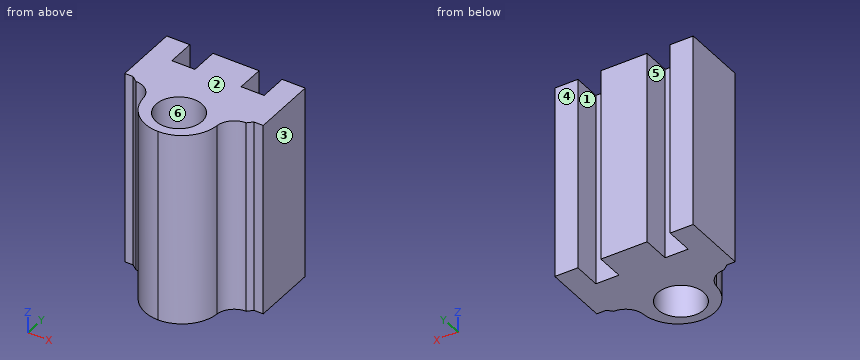
from build123d import *

# Parameters (mm, degrees)
SKETCH1_W           = 60
SKETCH1_H           = 42
BOSS_EXTRUDE1_DEPTH = 8
SKETCH3_W           = 10
SKETCH3_H           = 42
BOSS_EXTRUDE5_DEPTH = 6
SKETCH5_W           = 14
SKETCH5_H           = 42
BOSS_EXTRUDE6_DEPTH = 11
SKETCH6_R           = 5
CUT_EXTRUDE1_DEPTH  = 75.565407529
FILLET1_R           = 7
FILLET2_R           = 5
FILLET3_R           = 5
BOSS_EXTRUDE7_DEPTH = 42
SKETCH9_W           = 5
SKETCH9_H           = 42
BOSS_EXTRUDE8_DEPTH = 6
SKETCH11_W          = 15
SKETCH11_H          = 42
CUT_EXTRUDE2_DEPTH  = 76.921011584


with BuildPart() as part:
    # Sketch1 → Boss-Extrude1 (new body)
    with BuildSketch(Plane(origin=(0, 0, 0), x_dir=(1, 0, 0), z_dir=(0, 1, 0))):
        with Locations((30, 21)):
            Rectangle(SKETCH1_W, SKETCH1_H)
    extrude(amount=BOSS_EXTRUDE1_DEPTH)

    # Sketch3 → Boss-Extrude5 (add)
    with BuildSketch(Plane(origin=(0, 8, 0), x_dir=(1, 0, 0), z_dir=(0, 1, 0))):
        with Locations((30, 21)):
            Rectangle(SKETCH3_W, SKETCH3_H)
    extrude(amount=BOSS_EXTRUDE5_DEPTH)

    # Sketch5 → Boss-Extrude6 (add)
    with BuildSketch(Plane.XZ):
        with Locations((30, -21)):
            Rectangle(SKETCH5_W, SKETCH5_H)
    extrude(amount=BOSS_EXTRUDE6_DEPTH)

    # Sketch6 → Cut-Extrude1 (cut, through all)
    with BuildSketch(Plane(origin=(0, 0, -42), x_dir=(-1, 0, 0), z_dir=(0, 0, -1))):
        with Locations((-30, -5)):
            Circle(SKETCH6_R)
    extrude(amount=-CUT_EXTRUDE1_DEPTH, mode=Mode.SUBTRACT)

    # Fillet1
    fillet1_edges = [part.edges().sort_by_distance(p)[0] for p in [
        (23, -11, -21),
        (37, -11, -21),
    ]]
    fillet(fillet1_edges, radius=FILLET1_R - 0.0001)  # a hair under: the kernel refuses the full size

    # Fillet2
    fillet2_edges = [part.edges().sort_by_distance(p)[0] for p in [
        (23, 0, -21),
    ]]
    fillet(fillet2_edges, radius=FILLET2_R)

    # Fillet3
    fillet3_edges = [part.edges().sort_by_distance(p)[0] for p in [
        (37, 0, -21),
    ]]
    fillet(fillet3_edges, radius=FILLET3_R)

    # Sketch8 → Boss-Extrude7 (add)
    with BuildSketch(Plane(origin=(0, 0, -42), x_dir=(-1, 0, 0), z_dir=(0, 0, -1))):
        with BuildLine():
            Line((-41.958260743, -1), (-42.958260743, 0))
            Line((-42.958260743, 0), (-41.958260743, 0))
            ThreePointArc((-41.958260743, 0), (-38.573244741, -1.320099639), (-36.9756521, -4.583333333))
            ThreePointArc((-36.9756521, -4.583333333), (-34.739022403, -9.151860505), (-30, -11))
            ThreePointArc((-30, -11), (-25.260977597, -9.151860505), (-23.0243479, -4.583333333))
            ThreePointArc((-23.0243479, -4.583333333), (-21.426755259, -1.320099639), (-18.041739257, 0))
            Line((-18.041739257, 0), (-16.803044796, 0))
            Line((-16.803044796, 0), (-18.041739257, -1))
            ThreePointArc((-18.041739257, -1), (-20.749752058, -2.056079711), (-22.027826171, -4.666666667))
            ThreePointArc((-22.027826171, -4.666666667), (-24.583974397, -9.887840578), (-30, -12))
            ThreePointArc((-30, -12), (-35.416025603, -9.887840578), (-37.972173829, -4.666666667))
            ThreePointArc((-37.972173829, -4.666666667), (-39.250247942, -2.056079711), (-41.958260743, -1))
        make_face()
    extrude(amount=-BOSS_EXTRUDE7_DEPTH)

    # Sketch9 → Boss-Extrude8 (add)
    with BuildSketch(Plane(origin=(0, 8, 0), x_dir=(1, 0, 0), z_dir=(0, 1, 0))):
        with Locations((42.5, 21)):
            Rectangle(SKETCH9_W, SKETCH9_H)
        with Locations((17.5, 21)):
            Rectangle(SKETCH9_W, SKETCH9_H)
    extrude(amount=BOSS_EXTRUDE8_DEPTH)

    # Sketch11 → Cut-Extrude2 (cut, through all)
    with BuildSketch(Plane(origin=(0, 8, 0), x_dir=(1, 0, 0), z_dir=(0, 1, 0))):
        with Locations((52.5, 21)):
            Rectangle(SKETCH11_W, SKETCH11_H)
        with Locations((7.5, 21)):
            Rectangle(SKETCH11_W, SKETCH11_H)
    extrude(amount=-CUT_EXTRUDE2_DEPTH, mode=Mode.SUBTRACT)


solid = part.part
Design review of the part built by this model. Coordinates are the model's own, in mm. Face numbers are marked on the shaded views. A direction names the side the tool comes from. Coordinates: 2 decimals unless noted, no trailing zeros. Loops run counter-clockwise (first coordinate to the right, second up) from the corner with the lowest first, then second, coordinate; pieces in that order, holes last. Notation, with made-up numbers: (63.5, 27) -> (111.5, 27) arc R23 cw to (111.5, 63) -> close; hole circle Ø7 at (4.25, 30.5). An arc over 180 degrees is marked (long way). Use a Markdown table: item, result. Add a question column.
Item 1: We need section C-C, the plane x = 28.5. Write out the cut boundary in (y, z).
Item 2: Clearance check with flat-ended pins moving along their axes: P1, Ø2, axis at x = 38, z = -22.5, coming from the -Y side; P2, Ø4, axis at x = 37.5, z = -18, coming from the +Y side; P3, Ø2, axis at x = 16, z = -27.5, coming from the -Y side; P4, Ø6, axis at x = 30, y = -5, coming from the +Z side. State where each tip first meets the part, or that it passes through.
Item 3: Machinability: for the marked faces 1 and 2, which of the approach directions +Z, -Z, +X, -X, +Y, -Y give a long, thin tool a straight path to every point of the face, cutting with its end or side? Answer none if there is none.
Item 4: The part is to be moulded in two halves that separate along X. For the marked faces 3, 4, 5 and 6, say which applies: +X half, -X half, draft (parallel to the pull), parting line (faces both ways), or undercut.
Item 5: We need section D-D, the plane y = -6.5. Write out the cut boundary in (x, z), and give its area (3 significant figures).
Item 6: We need section B-B, the plane z = -20. Write out the cut boundary in (x, y), and give its area (3 significant figures).
Item 7: Wall thickness on L1, parallel to X at y = 11.5, z = -37; L2, parallel to Y at x = 30, z = -20.5; L3, parallel to X at y = -2.5, z = -28.5: over which ranges is each line inside the solid? List them lowest first. Write a range as from..to.
Item 8: We need section A-A, the plane y = 9.5. Write out the cut boundary in (x, z), and give its area (3 significant figures).
Numbers:
| question | item | result |
|---|---|---|
| 1 | outline | (-11.86, -42) -> (-9.77, -42) -> (-9.77, 0) -> (-11.86, 0) -> close; (-0.23, -42) -> (14, -42) -> (14, 0) -> (-0.23, 0) -> close |
| 2 | P1 | stops at y = -7.87 |
| 2 | P2 | stops at y = 8 |
| 2 | P3 | stops at y = -0.16 |
| 2 | P4 | passes through |
| 3 | face 1 | +Z, -Z, +Y |
| 3 | face 2 | +Z, +X, -X, +Y, -Y |
| 4 | face 3 | +X half |
| 4 | face 4 | draft |
| 4 | face 5 | undercut |
| 4 | face 6 | undercut |
| 5 | outline | (22.4, -42) -> (25.23, -42) -> (25.23, 0) -> (22.4, 0) -> close; (34.77, -42) -> (37.6, -42) -> (37.6, 0) -> (34.77, 0) -> close |
| 5 | area | 238 mm^2 |
| 6 | outline | (15, 0) -> (16.8, 0) -> (18.04, -1) arc R4 cw to (22.03, -4.67) arc R8 ccw to (37.97, -4.67) arc R4 cw to (41.96, -1) -> (42.96, 0) -> (45, 0) -> (45, 14) -> (40, 14) -> (40, 8) -> (35, 8) -> (35, 14) -> (25, 14) -> (25, 8) -> (20, 8) -> (20, 14) -> (15, 14) -> close; hole circle Ø10 at (30, -5) |
| 6 | area | 462 mm^2 |
| 7 | L1 | x = 15..20, 25..35, 40..45 |
| 7 | L2 | y = -12..-10, 0..14 |
| 7 | L3 | x = 21.16..25.67, 34.33..38.84 |
| 8 | outline | (15, -42) -> (20, -42) -> (20, 0) -> (15, 0) -> close; (25, -42) -> (35, -42) -> (35, 0) -> (25, 0) -> close; (40, -42) -> (45, -42) -> (45, 0) -> (40, 0) -> close |
| 8 | area | 840 mm^2 |
